Work out the finished part from the listing and answer in its coordinate system (mm). Coordinates: 2 decimals unless noted, no trailing zeros. Write each loop counter-clockwise with the first axis right and the second up, starting at its lowest first coordinate (ties: lowest second). Pieces come first, ordered by that corner, then holes. Notation, with made-up numbers: (-2.5, -35.75) - (46.5, -35.75) arc R29 ccw to (46.5, -4.75) - close; hole circle Ø8 at (-32, -14). An arc over 180 degrees is marked (long way). Use one line per item in the form item = value. Start each with the question number.
Item 1: A cutting plane is placed at A-A (y = -106.5). Write down the section's boundary in (x, z), then the cut area to 3 significant figures.
Item 2: Consider probe 1 along Y at (x, z) = (0, 1.9); probe 2 along X at (y, z) = (1.5, 3.85); probe 3 along X at (y, z) = (-143, 3). Determine where each line is inside the solid, lowest interval first.
Item 3: Given pin 1 (1.5 mm diameter, centred on y = -123, z = 3, fed in from +X); pin 2 (3.5 mm diameter, centred on x = 0, y = -41.37, fed in from +Z); pin 3 (1 mm diameter, centred on x = 112, z = 4, fed in from -Y); pin 4 (3 mm diameter, centred on x = -54, z = 1, fed in from -Y), each flat-ended and moving along its own axis, determine where each tip first touches the part or whether it passes through.
Item 4: A cutting plane is placed at C-C (x = -142.5). Write down the section's boundary in (y, z), then the cut area to 3 significant figures.
Item 5: A cutting plane is placed at D-D (z = 0.8). Give the number of separate pieces and of enclosed holes in the cut face, then the cut area to 3 significant figures.
Item 6: A cutting plane is placed at B-B (y = 33). Write down the section's boundary in (x, z), then the cut area to 3 significant figures.
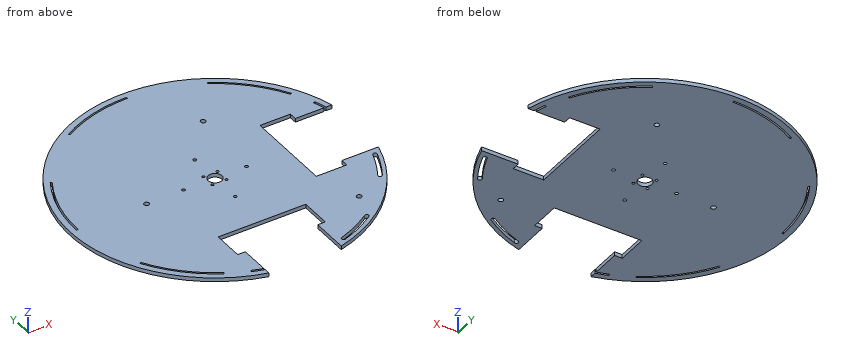
from build123d import *

# Parameters (mm, degrees)
SKETCH1_R           = 3.25
SKETCH1_R_2         = 2.1
SKETCH1_R_3         = 1.75
SKETCH1_R_4         = 9
BOSS_EXTRUDE1_DEPTH = 5


with BuildPart() as part:
    # Sketch1 → Boss-Extrude1 (new body)
    with BuildSketch(Plane.XY):
        with BuildLine():
            Line((47.5, -135.966708945), (47.5, -183.966708945))
            ThreePointArc((47.5, -183.966708945), (134.350288425, -134.350288425), (183.966708945, -47.5))
            Line((183.966708945, -47.5), (135.966708945, -47.5))
            Line((135.966708945, -47.5), (135.966708945, -57.5))
            Line((135.966708945, -57.5), (95.966708945, -57.5))
            Line((95.966708945, -57.5), (95.966708945, 57.5))
            Line((95.966708945, 57.5), (135.966708945, 57.5))
            Line((135.966708945, 57.5), (135.966708945, 47.5))
            Line((135.966708945, 47.5), (173.61955535, 47.5))
            ThreePointArc((173.61955535, 47.5), (171.490271693, 54.690828433), (169.063304941, 61.786721248))
            Line((169.063304941, 61.786721248), (171.411406398, 62.644870154))
            ThreePointArc((171.411406398, 62.644870154), (173.97563055, 55.124676642), (176.210101867, 47.5))
            Line((176.210101867, 47.5), (183.966708945, 47.5))
            ThreePointArc((183.966708945, 47.5), (-134.350288425, 134.350288425), (-47.5, -183.966708945))
            Line((-47.5, -183.966708945), (-47.5, -176.210101867))
            ThreePointArc((-47.5, -176.210101867), (-55.124676642, -173.97563055), (-62.644870154, -171.411406398))
            Line((-62.644870154, -171.411406398), (-61.786721248, -169.063304941))
            ThreePointArc((-61.786721248, -169.063304941), (-54.690828433, -171.490271693), (-47.5, -173.61955535))
            Line((-47.5, -173.61955535), (-47.5, -135.966708945))
            Line((-47.5, -135.966708945), (-57.5, -135.966708945))
            Line((-57.5, -135.966708945), (-57.5, -95.966708945))
            Line((-57.5, -95.966708945), (57.5, -95.966708945))
            Line((57.5, -95.966708945), (57.5, -135.966708945))
            Line((57.5, -135.966708945), (47.5, -135.966708945))
        make_face()
        with Locations((47.553086042, 98.224543307)):
            Circle(SKETCH1_R, mode=Mode.SUBTRACT)
        with BuildLine():
            Line((-90.06771897, 155.845455499), (-91.168546646, 157.750233288))
            ThreePointArc((-91.168546646, 157.750233288), (-46.86549419, 176.069490413), (0.682251823, 182.198722642))
            Line((0.682251823, 182.198722642), (0.674013875, 179.998738066))
            ThreePointArc((0.674013875, 179.998738066), (-46.299610067, 173.943514129), (-90.06771897, 155.845455499))
        make_face(mode=Mode.SUBTRACT)
        with BuildLine():
            ThreePointArc((-155.845455499, 90.06771897), (-173.943514129, 46.299610067), (-179.998738066, -0.674013875))
            Line((-179.998738066, -0.674013875), (-182.198722642, -0.682251823))
            ThreePointArc((-182.198722642, -0.682251823), (-176.069490413, 46.86549419), (-157.750233288, 91.168546646))
            Line((-157.750233288, 91.168546646), (-155.845455499, 90.06771897))
        make_face(mode=Mode.SUBTRACT)
        with BuildLine():
            Line((-88.977505429, -156.470455766), (-90.065008273, -158.382872448))
            ThreePointArc((-90.065008273, -158.382872448), (-128.259298986, -129.407852249), (-157.573663687, -91.473386907))
            Line((-157.573663687, -91.473386907), (-155.671017912, -90.368878394))
            ThreePointArc((-155.671017912, -90.368878394), (-126.710613707, -127.845298599), (-88.977505429, -156.470455766))
        make_face(mode=Mode.SUBTRACT)
        with Locations((-89.999369033, -0.337006938)):
            Circle(SKETCH1_R, mode=Mode.SUBTRACT)
        with Locations((-41.37, 0)):
            Circle(SKETCH1_R_2, mode=Mode.SUBTRACT)
        with Locations((-9.192388155, -9.192388155)):
            Circle(SKETCH1_R_3, mode=Mode.SUBTRACT)
        with BuildLine():
            ThreePointArc((103.668630414, -153.224720813), (81.760900425, -165.952267721), (58.319627193, -175.567141243))
            ThreePointArc((58.319627193, -175.567141243), (55.032569907, -173.919338342), (56.680372807, -170.632281056))
            ThreePointArc((56.680372807, -170.632281056), (79.462756197, -161.287663439), (100.754701342, -148.917863795))
            ThreePointArc((100.754701342, -148.917863795), (104.365094387, -149.614327769), (103.668630414, -153.224720813))
        make_face(mode=Mode.SUBTRACT)
        with Locations((115.206196365, -115.206196365)):
            Circle(SKETCH1_R, mode=Mode.SUBTRACT)
        with Locations((0, -41.37)):
            Circle(SKETCH1_R_2, mode=Mode.SUBTRACT)
        with Locations((9.192388155, -9.192388155)):
            Circle(SKETCH1_R_3, mode=Mode.SUBTRACT)
        Circle(SKETCH1_R_4, mode=Mode.SUBTRACT)
        with Locations((41.37, 0)):
            Circle(SKETCH1_R_2, mode=Mode.SUBTRACT)
        with BuildLine():
            ThreePointArc((175.567141243, -58.319627193), (168.13089268, -77.181622984), (158.67524262, -95.116598864))
            ThreePointArc((158.67524262, -95.116598864), (155.108438361, -96.009855479), (154.215181746, -92.443051221))
            ThreePointArc((154.215181746, -92.443051221), (163.405051373, -75.012193581), (170.632281056, -56.680372807))
            ThreePointArc((170.632281056, -56.680372807), (173.919338342, -55.032569907), (175.567141243, -58.319627193))
        make_face(mode=Mode.SUBTRACT)
        with Locations((-9.192388155, 9.192388155)):
            Circle(SKETCH1_R_3, mode=Mode.SUBTRACT)
        with Locations((9.192388155, 9.192388155)):
            Circle(SKETCH1_R_3, mode=Mode.SUBTRACT)
        with Locations((0, 41.37)):
            Circle(SKETCH1_R_2, mode=Mode.SUBTRACT)
        with BuildLine():
            ThreePointArc((91.473386907, 157.573663687), (129.407852249, 128.259298986), (158.382872448, 90.065008273))
            Line((158.382872448, 90.065008273), (156.470455766, 88.977505429))
            ThreePointArc((156.470455766, 88.977505429), (127.845298599, 126.710613707), (90.368878394, 155.671017912))
            Line((90.368878394, 155.671017912), (91.473386907, 157.573663687))
        make_face(mode=Mode.SUBTRACT)
    extrude(amount=BOSS_EXTRUDE1_DEPTH)


solid = part.part
Answer:
q1.outline = (-157.35, 0) - (-147.83, 0) - (-147.83, 5) - (-157.35, 5) - close; (-145.11, 0) - (-57.5, 0) - (-57.5, 5) - (-145.11, 5) - close; (57.5, 0) - (157.35, 0) - (157.35, 5) - (57.5, 5) - close
q1.area = 985 mm²
q2.probe_1 = -95.97 to -43.47, -39.27 to -9, 9 to 39.27, 43.47 to 180, 182.2 to 190
q2.probe_2 = -189.99 to -182.19, -179.99 to -92.68, -87.32 to -42.84, -39.9 to -8.87, 8.87 to 39.9, 42.84 to 95.97
q2.probe_3 = -125.1 to -112.91, -109.32 to -47.5, 47.5 to 125.1
q3.pin_1 = 145.45
q3.pin_2 = through
q3.pin_3 = -153.84
q3.pin_4 = -182.6
q4.outline = (-125.67, 0) - (-113.54, 0) - (-113.54, 5) - (-125.67, 5) - close; (-109.97, 0) - (125.67, 0) - (125.67, 5) - (-109.97, 5) - close
q4.area = 1,240 mm²
q5.separate_pieces = 1
q5.enclosed_holes = 18
q5.area = 92,400 mm²
q6.outline = (-187.11, 0) - (-179.19, 0) - (-179.19, 5) - (-187.11, 5) - close; (-176.95, 0) - (95.97, 0) - (95.97, 5) - (-176.95, 5) - close
q6.area = 1,400 mm²
